Geometry check sheet. Reference: drawing and pictorial views, mm from the part's lowest x, y, z. A direction names the side the tool comes from. Round coordinates to 2 decimals unless told otherwise and drop trailing zeros. Order: outer loops, then holes, each group sorted by start corner. A loop starts at its lowest first (then second) coordinate and runs counter-clockwise, first axis right, second up.
(1) Sectioned sample at D-D (y = 29). Record the boundary of the cut face in (x, z), plus the area to 3 significant figures.
(2) Material ranges on line 1 along Z through (x, y) = (13.5, 36.25) (1 decimal); line 2 along Y through (x, z) = (4, 18.5); line 3 along Z through (x, y) = (13, 35), recorded low to high.
(3) Sectioned sample at B-B (z = 21). Record the boundary of the cut face in (x, y), plus the area to 3 significant figures.
(4) Set-up check for the marked faces 1 and 2: record each of +Z, -Z, +X, -X, +Y, -Y from which the full face is reachable in a straight line by a thin tool's end or side.
(5) Go/stop test with flat-tipped pins: pin 1 (4 mm diameter, centred on x = 28.5, z = 8.01, fed in from -Y); pin 2 (2 mm diameter, centred on x = 23.5, y = 12.5, fed in from +Z); pin 3 (6 mm diameter, centred on y = 7.5, z = 20, fed in from +X); pin 4 (4 mm diameter, centred on x = 21, z = 21, fed in from +Y). Record where each tip stops, or that it passes through.
(6) Sectioned sample at C-C (z = 35). Record the boundary of the cut face in (x, y), plus the area to 3 significant figures.
(7) Sectioned sample at A-A (x = 21). Record the boundary of the cut face in (y, z).
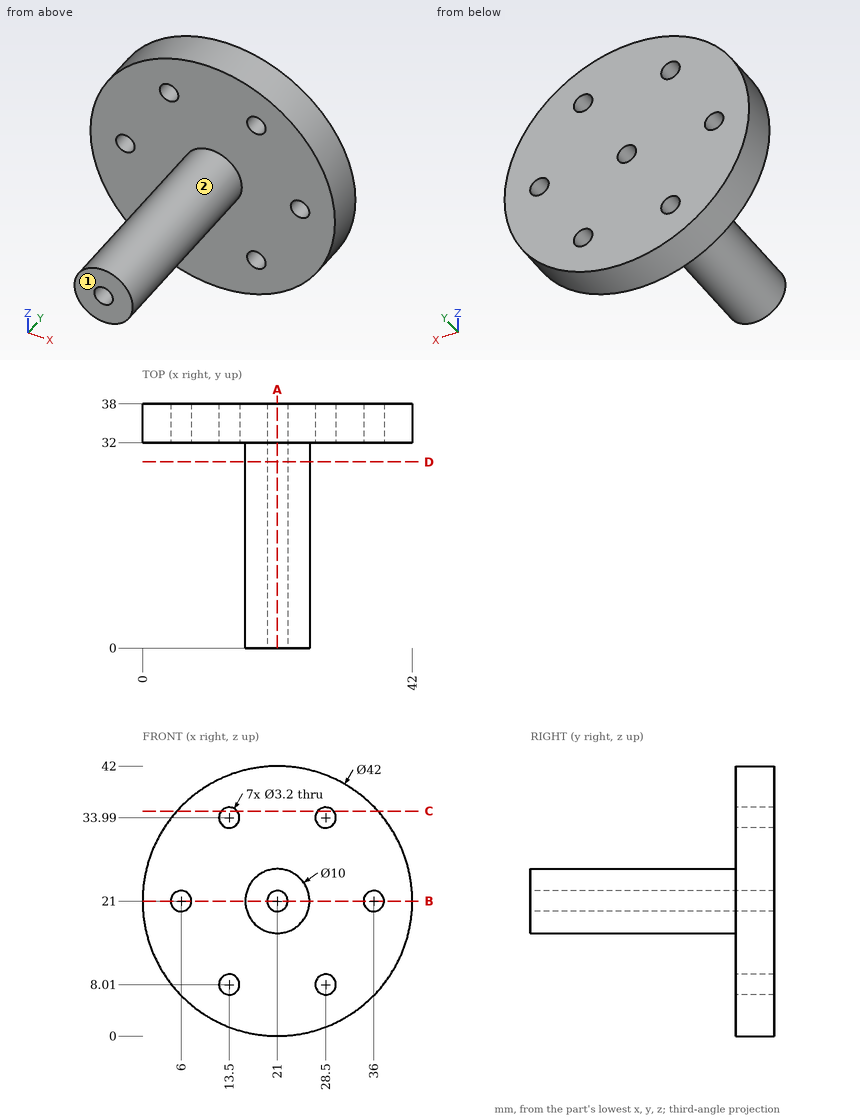
Answer below:
1. outline: circle Ø10 at (21, 21); hole circle Ø3.2 at (21, 21)
1. area: 70.5 mm2
2. line 1: z = 1.4 to 6.4, 9.6 to 32.4, 35.6 to 40.6
2. line 2: y = 32 to 38
2. line 3: z = 1.58 to 6.49, 9.53 to 32.47, 35.51 to 40.42
3. outline: (0, 32) - (4.4, 32) - (4.4, 38) - (0, 38) - close; (7.6, 32) - (16, 32) - (16, 0) - (19.4, 0) - (19.4, 38) - (7.6, 38) - close; (22.6, 0) - (26, 0) - (26, 32) - (34.4, 32) - (34.4, 38) - (22.6, 38) - close; (37.6, 32) - (42, 32) - (42, 38) - (37.6, 38) - close
3. area: 412 mm2
4. face 1: +Z, -Z, +X, -X, -Y
4. face 2: -Y
5. pin 1: stops at y = 32
5. pin 2: stops at z = 25.77
5. pin 3: stops at x = 26
5. pin 4: stops at y = 38
6. outline: (5.35, 32) - (12.26, 32) - (12.26, 38) - (5.35, 38) - close; (14.74, 32) - (27.26, 32) - (27.26, 38) - (14.74, 38) - close; (29.74, 32) - (36.65, 32) - (36.65, 38) - (29.74, 38) - close
6. area: 158 mm2
7. outline: (0, 16) - (32, 16) - (32, 0) - (38, 0) - (38, 19.4) - (0, 19.4) - close; (0, 22.6) - (38, 22.6) - (38, 42) - (32, 42) - (32, 26) - (0, 26) - close
